Geometry: final body of the model. Coordinates: model frame, mm. Face numbers are marked on the shaded views. Give positions to 0.01 mm unless a question says otherwise; leave off trailing zeros. Write each loop counter-clockwise with the first axis right and the second up, starting at its lowest first coordinate (ties: lowest second). Pieces come first, ordered by that corner, then holes. Notation, with made-up numbers: M -12.5,56.25 L 19.5,56.25 A25 cw 19.5,74.25 Z; hole C 77.5,10.25 d9. An arc over 180 degrees is marked long. Use a Markdown table: item, result. Add a question column.
1) Pin query (flat end, axial travel): pin 1 (1 mm diameter, centred on x = 5, z = 5.5, fed in from +Y). Return the tip coordinate at first contact, or that it passes through.
2) Section C-C on y = -15. Return the cut outline in (x, z), then the cut area to 3 significant figures.
3) Section A-A on y = -8. Return the cut outline in (x, z).
4) Draft query along X for the marked faces 1, 2, 3 and 4. Return one class per face: +X half, -X half, draft (parallel to the pull), parting line (faces both ways), or undercut.
5) Section B-B on x = 5.75. Return the cut outline in (y, z), then the cut area to 3 significant figures.
6) Section D-D on z = 3.75. State how many separate pieces and enclosed holes the cut face has, then the cut area to 3 significant figures.
7) Line query: line 1 (X direction, y = -4, z = 2); line 2 (X direction, y = -13, z = 6); line 3 (Z direction, x = 6.45, y = -15). Output: solid intervals per line, ascending.
```python
from build123d import *

# Parameters (mm, degrees)
F0_W        = 8
F0_H        = 8
F1_DEPTH    = 20
F2_R        = 3.99999
F4_DEPTH    = 25
F6_T1_DEPTH = 27.364916731
F5_R        = 2.5
F7_DEPTH    = 25


# Not quite as in the source:
# - a fillet or chamfer that OpenCascade refuses, or shapes differently, is made with other operations: its cross-section is extruded or revolved along the edge and cut away or added
# - a fillet or chamfer is up to 0.001 mm smaller than in the source, because OpenCascade refuses the exact size


with BuildPart() as f1:
    # F0 (on Front) → F1 (new body)
    with BuildSketch(Plane.XZ):
        with Locations((4, 4)):
            Rectangle(F0_W, F0_H)
    extrude(amount=F1_DEPTH)

    # F2 (radius 4 in the source; OpenCascade refuses exactly that, so slightly less here)
    f2_edges = [f1.edges().sort_by_distance(p)[0] for p in [
        (8, 0, 4),
        (0, 0, 4),
    ]]
    fillet(f2_edges, radius=F2_R)

    # F3 (on face) → F4 (cut)
    with BuildSketch(Plane.XY.offset(8)):
        with BuildLine():
            Line((5, -20), (5, -6.5617376915))
            ThreePointArc((5, -6.5617376915), (4, -1.25), (3, -6.5617376915))
            Line((3, -6.5617376915), (3, -20))
            Line((3, -20), (4, -20))
            Line((4, -20), (5, -20))
        make_face()
    extrude(amount=-F4_DEPTH, mode=Mode.SUBTRACT)

    # F6: fillet of radius 4 on 2 edges, made by hand

    # F6_s2 → F6_t1 (cut)
    with BuildSketch(Plane.XY.offset(-9.6824583655)):
        with BuildLine():
            ThreePointArc((0, -16.1270166538), (0.8377223398, -18.5765063966), (3, -20))
            Line((3, -20), (0, -20))
            Line((0, -20), (0, -16.1270166538))
        make_face()
        with BuildLine():
            ThreePointArc((5, -20), (7.1622776602, -18.5765063966), (8, -16.1270166538))
            Line((8, -16.1270166538), (8, -20))
            Line((8, -20), (5, -20))
        make_face()
    extrude(amount=F6_T1_DEPTH, mode=Mode.SUBTRACT)

    # F5 (on face) → F7 (cut)
    with BuildSketch(Plane(origin=(0, 0, 0), x_dir=(0, -1, 0), z_dir=(-1, 0, 0))):
        with Locations((15, 4)):
            Circle(F5_R)
    extrude(amount=-F7_DEPTH, mode=Mode.SUBTRACT)


solid = f1.part
```
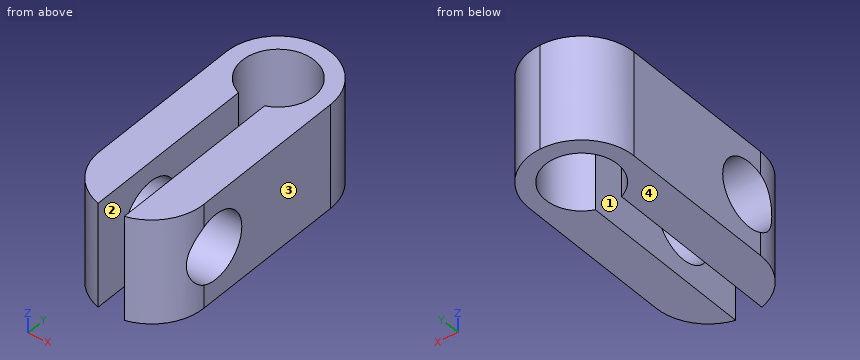
Found:
| question | item | result |
|---|---|---|
| 1 | pin 1 | y = -0.03 |
| 2 | outline | M 0,0 L 3,0 L 3,1.5 L 0,1.5 Z; M 0,6.5 L 3,6.5 L 3,8 L 0,8 Z; M 5,0 L 8,0 L 8,1.5 L 5,1.5 Z; M 5,6.5 L 8,6.5 L 8,8 L 5,8 Z |
| 2 | area | 18.0 mm² |
| 3 | outline | M 0,0 L 3,0 L 3,8 L 0,8 Z; M 5,0 L 8,0 L 8,8 L 5,8 Z |
| 4 | face 1 | undercut |
| 4 | face 2 | undercut |
| 4 | face 3 | +X half |
| 4 | face 4 | draft |
| 5 | outline | M -19.72,0 L -6.12,0 L -6.12,8 L -19.72,8 Z; M -1.88,0 L -0.4,0 L -0.4,8 L -1.88,8 Z; hole C -15,4 d5 |
| 5 | area | 101 mm² |
| 6 | separate pieces | 3 |
| 6 | enclosed holes | 0 |
| 6 | area | 67.1 mm² |
| 7 | line 1 | 0 to 1.25, 6.75 to 8 |
| 7 | line 2 | 0 to 3, 5 to 8 |
| 7 | line 3 | 0 to 1.5, 6.5 to 8 |
